from build123d import *

# Parameters (mm, degrees)
F0_W           = 90
F0_H           = 45
F1_DEPTH       = 12
F2_R           = 6.5
F2_R_2         = 10
F3_DEPTH       = 25
F4_SIZE        = 0.8
F7_D           = 6
F7_CSINK_D     = 8
F7_CSINK_ANGLE = 90
F9_D           = 4
F9_DEPTH       = 30
F9_CSINK_D     = 5
F9_CSINK_ANGLE = 90
F9_TIP         = 1.2017212381


with BuildPart() as f1:
    # F0 (on Front) → F1 (new body)
    with BuildSketch(Plane.XZ):
        Rectangle(F0_W, F0_H)
    extrude(amount=-F1_DEPTH)

    # F2 (on Front) → F3 (cut)
    with BuildSketch(Plane.XZ):
        with Locations((-20, 0)):
            Circle(F2_R)
        with Locations((20, 0)):
            Circle(F2_R_2)
    extrude(amount=-F3_DEPTH, mode=Mode.SUBTRACT)

    # F4
    f4_edges = [f1.edges().sort_by_distance(p)[0] for p in [
        (-26.5, 0, 0),
        (-26.5, 12, 0),
        (10, 0, 0),
        (10, 12, 0),
    ]]
    chamfer(f4_edges, length=F4_SIZE)

    # F7 (through all)
    with Locations(Plane.XY.offset(22.5)):
        with Locations((-39, 6), (39, 6)):
            CounterSinkHole(F7_D / 2, F7_CSINK_D / 2, counter_sink_angle=F7_CSINK_ANGLE)

    # F9
    with Locations(Plane.YZ.offset(45)):
        with Locations((6, 0)):
            CounterSinkHole(F9_D / 2, F9_CSINK_D / 2, depth=F9_DEPTH, counter_sink_angle=F9_CSINK_ANGLE)
            with Locations((0, 0, -(F9_DEPTH + F9_TIP / 2))):  # 118° drill point
                Cone(0, F9_D / 2, F9_TIP, mode=Mode.SUBTRACT)


solid = f1.part
Check sheet for the modelled part. Datum: model origin and axes. Units: mm. A direction names the side the tool comes from. Round coordinates to 2 decimals unless told otherwise and drop trailing zeros. Write each loop counter-clockwise with the first axis right and the second up, starting at its lowest first coordinate (ties: lowest second). Pieces come first, ordered by that corner, then holes. Notation, with made-up numbers: (35.25, 71.5) -> (70.25, 71.5) arc R22 cw to (70.25, 87.5) -> close; hole circle Ø6 at (-4.5, 28). An arc over 180 degrees is marked (long way). Answer as CSV lines item,"result". Start each with the question number.
1) Tool access check on faces 1 (the cylindrical face through (43.208, 4.153, -0.766)), 2 (the cylindrical face through (39, 9, -1)). Record the directions out of +Z, -Z, +X, -X, +Y, -Y that give a thin tool (end or side, any length) a straight path to the whole face; none if there is none.
2) Section check A-A on z = 0. State how many separate pieces and enclosed holes the cut face has, and give its area (3 significant figures).
3) Release check for a two-part mould opening along Y. For faces 3 (the cylindrical face through (33, 8, 0)), 4 (the cylindrical face through (-36, 6, -1)), 5 (the cylindrical face through (-26.494, 5.927, 0.286)), 6 (the flat face through (-1, 12, 0)) record: pulls with the +Y half, pulls with the -Y half, needs draft (parallel to the pull), parting line crosses it, or undercut.
4) Material ranges on line 1 (X direction, y = 8.25, z = 17); line 2 (Y direction, x = -39, z = 2); line 3 (X direction, y = 8, z = -18), recorded low to high. Write a range as from..to.
5) Section check C-C on y = 6. Enter the section's corners in (x, z).
6) Section check D-D on z = -17. Enter the section's corners in (x, y).
7) Section check B-B on x = 20. Enter the section's corners in (y, z), and give its area (3 significant figures).
Found:
1,face 1,"+X"
1,face 2,"+Z, -Z"
2,separate pieces,"4"
2,enclosed holes,"1"
2,area,"587 mm^2"
3,face 3,"undercut"
3,face 4,"undercut"
3,face 5,"needs draft"
3,face 6,"pulls with the +Y half"
4,line 1,"x = -45..-40.98, -37.02..37.02, 40.98..45"
4,line 2,"y = 0..3, 9..12"
4,line 3,"x = -45..-41.24, -36.76..36.76, 41.24..45"
5,outline,"(-45, -22.5) -> (-42, -22.5) -> (-42, 21.5) -> (-43, 22.5) -> (-45, 22.5) -> close; (-36, -22.5) -> (36, -22.5) -> (36, -2) -> (29.8, -2) arc R10 cw (long way) to (29.8, 2) -> (36, 2) -> (36, 21.5) -> (35, 22.5) -> (-35, 22.5) -> (-36, 21.5) -> close; (42, -22.5) -> (45, -22.5) -> (45, -2.5) -> (44.5, -2) -> (42, -2) -> close; (42, 2) -> (44.5, 2) -> (45, 2.5) -> (45, 22.5) -> (43, 22.5) -> (42, 21.5) -> close; hole circle Ø13 at (-20, 0)"
6,outline,"(-45, 0) -> (45, 0) -> (45, 12) -> (-45, 12) -> close; hole circle Ø6 at (-39, 6); hole circle Ø6 at (39, 6)"
7,outline,"(0, -22.5) -> (12, -22.5) -> (12, -10.8) -> (11.2, -10) -> (0.8, -10) -> (0, -10.8) -> close; (0, 10.8) -> (0.8, 10) -> (11.2, 10) -> (12, 10.8) -> (12, 22.5) -> (0, 22.5) -> close"
7,area,"299 mm^2"
